For this review, take the finished solid that the model builds, in its own axes (mm). A direction names the side the tool comes from. Round coordinates to 2 decimals unless told otherwise and drop trailing zeros. Loops run counter-clockwise (first coordinate to the right, second up) from the corner with the lowest first, then second, coordinate; pieces in that order, holes last.
```python
from build123d import *

# Parameters (mm, degrees)
F2_R            = 12.7
F3_DEPTH        = 30.1635
F3_COPIES_COUNT = 12
F4_R            = 3.175
F5_SIZE2        = 2.286
F5_SIZE         = 2.286


# Not quite as in the source:
# - a pattern or mirror of a feature is missing from the dataset's text; its kind, count and spacing are read off the source's solid


with BuildPart() as f1:
    # F0 (on Front) → F1 (revolve)
    with BuildSketch(Plane.XZ):
        Polygon((-101.6, 127.254), (0, 127.254), (0, 161.925), (-1.5875, 161.925), (-1.5875, 203.2), (-30.1625, 203.2), (-30.1625, 152.4), (-54.61, 138.1125), (-95.25, 136.525), (-101.6, 128.8415), align=None)
    revolve(axis=Axis((-71.3775697505, 0, 0), (-1, 0, 0)))

    # F2 (on face) → F3 (cut, through all)
    with BuildSketch(Plane(origin=(-30.1625, 0, 0), x_dir=(0, -1, 0), z_dir=(-1, 0, 0))):
        with Locations((0, 180.975)):
            Circle(F2_R)
    f3 = extrude(amount=-F3_DEPTH, mode=Mode.SUBTRACT)

    # F3_copies: F3 ×12 about axis
    f3_copies_axis = Axis((0, 0, 0), (1, 0, 0))
    for i in range(1, F3_COPIES_COUNT):
        add(f3.rotate(f3_copies_axis, i * 360 / F3_COPIES_COUNT), mode=Mode.SUBTRACT)

    # F4
    f4_edges = [f1.edges().sort_by_distance(p)[0] for p in [
        (-30.1625, 0, -152.4),
        (-54.61, 0, -138.1125),
    ]]
    fillet(f4_edges, radius=F4_R)

    # F5
    f5_edges = [f1.edges().sort_by_distance(p)[0] for p in [
        (-1.5875, 0, -203.2),
        (-30.1625, 0, -203.2),
        (-15.875, 0, 203.2),
    ]]
    chamfer(f5_edges, length=F5_SIZE, length2=F5_SIZE2)


solid = f1.part
```
(1) Add section C-C (x = -85). Give the boundary of the cut face in (y, z).
(2) For faces 5 (the cylindrical face through (-16.1, -6.8, 191.7)), 6 (the flat face through (-1.588, 90, 135)), list the 3-axis set-ups (+Z, -Z, +X, -X, +Y, -Y) from which the entire face can be reached by the end or side of a thin tool; tool diameter is ignored.
(3) Add section A-A (z = 0). Give the number of separate pieces and of enclosed holes in the cut face, plus the area to 3 significant figures.
(4) The part is to be moulded in two halves that separate along Y. For faces 1 (the cylindrical face through (-16.075, -95.352, -144.997)), 2 (the conical face through (-1.698, 60.382, 191.742)), 3 (the flat face through (-101.6, 125, -29)), 4 (the cylindrical face through (-16.1, -191.7, -6.8)), say which applies: pulls with the +Y half, pulls with the -Y half, needs draft (parallel to the pull), parting line crosses it, or undercut.
(5) Insertion check: pin 1 Ø6 at (y, z) = (79.5, 147.5) entering from -X; pin 2 Ø5 at (x, y) = (-61, -128) entering from -Z; pin 3 Ø6 at (y, z) = (-55.5, 124) entering from -X. Each pin has a flat end and moves straight along its axis. Give the tip position at first contact, or say it passes through.
(6) For L1, parallel to Y at x = -14.75, z = 0 (3 decimals); L2, parallel to X at y = -159.5, z = 37; L3, parallel to Z at x = -97, y = -79, list the stretches that pass through material, from the lowest coordinate up.
Outcome:
1. outline: circle Ø273.85 at (0, 0); hole circle Ø254.51 at (0, 0)
2. face 5: +X, -X
2. face 6: +X
3. separate pieces: 4
3. enclosed holes: 0
3. area: 4,760 mm2
4. face 1: undercut
4. face 2: parting line crosses it
4. face 3: needs draft
4. face 4: undercut
5. pin 1: stops at x = -30.16
5. pin 2: stops at z = -57.07
5. pin 3: stops at x = -98.28
6. L1: y = -203.2 to -193.675, -168.275 to -127.254, 127.254 to 168.275, 193.675 to 203.2
6. L2: x = -30.16 to -1.59
6. L3: z = -108.74 to -99.76, 99.76 to 108.74
